Read the model definition and answer for the solid it produces. Units are mm, in the model's axes. Give positions to 0.01 mm unless a question says otherwise; leave off trailing zeros. Loops run counter-clockwise (first coordinate to the right, second up) from the corner with the lowest first, then second, coordinate; pieces in that order, holes last. Notation, with made-up numbers: (21, 3) -> (62, 3) arc R28 ccw to (62, 34) -> close; hole circle Ø8 at (43.25, 77). An arc over 180 degrees is marked (long way). One line per item, written item: value. Start each with the question number.
from build123d import *

# Parameters (mm, degrees)
F0_R     = 10.668
F0_R_2   = 8.255
F1_DEPTH = 914.4
F2_R     = 4.1275
F3_DEPTH = 25.4


with BuildPart() as f1:
    # F0 (on Front) → F1 (new body)
    with BuildSketch(Plane.XZ):
        Circle(F0_R)
        Circle(F0_R_2, mode=Mode.SUBTRACT)
    extrude(amount=F1_DEPTH)

    # F2 (on Top) → F3 (cut)
    with BuildSketch(Plane.XY):
        with Locations((0, -101.6)):
            Circle(F2_R)
        with Locations((0, -279.4)):
            Circle(F2_R)
        with Locations((0, -457.2)):
            Circle(F2_R)
        with Locations((0, -635)):
            Circle(F2_R)
        with Locations((0, -812.8)):
            Circle(F2_R)
    extrude(amount=F3_DEPTH, mode=Mode.SUBTRACT)


solid = f1.part
Item 1: Section C-C, the plane y = -859 is taken. Determine the outline of the cut face in (x, z) (3 decimals), plus the area to 3 significant figures.
Item 2: Section A-A, the plane x = 0 is taken. Determine the outline of the cut face in (y, z) (1 decimal), plus the area to 3 significant figures.
Item 3: Flat-ended cylindrical pins translate along their axes: pin 1 (1 mm diameter, centred on x = -3.5, z = -5.5, fed in from -Y); pin 2 (1 mm diameter, centred on x = 4.5, y = -630.5, fed in from -Z); pin 3 (2 mm diameter, centred on y = -575, z = -8, fed in from +X); pin 4 (1.5 mm diameter, centred on x = 7, y = -187.5, fed in from +Z). Find the tip coordinate at first contact, or state that the pin passes through.
Item 4: Determine the mould class of faces 1 (the cylindrical face through (7.874, -450.799, 2.48)), 2 (the flat face through (3, -914.4, -8)), 3 (the cylindrical face through (4.923, -450.799, -9.464)) for opening direction X: pulls with the +X half, pulls with the -X half, needs draft (parallel to the pull), parting line crosses it, or undercut.
Item 5: Section B-B, the plane z = 3.75 is taken. Determine the outline of the cut face in (x, y).
Item 6: Consider L1, parallel to Y at x = 0, z = 9.8; L2, parallel to Z at x = 1.5, y = -771.5; L3, parallel to X at y = -656, z = 1. Determine where each line is inside the solid, lowest interval first. Write a range as [from, to].
Computed values:
1. outline: circle Ø21.336 at (0, 0); hole circle Ø16.51 at (0, 0)
1. area: 143 mm²
2. outline: (-914.4, -10.7) -> (0, -10.7) -> (0, -8.3) -> (-914.4, -8.3) -> close; (-914.4, 8.3) -> (-816.9, 8.3) -> (-816.9, 10.7) -> (-914.4, 10.7) -> close; (-808.7, 8.3) -> (-639.1, 8.3) -> (-639.1, 10.7) -> (-808.7, 10.7) -> close; (-630.9, 8.3) -> (-461.3, 8.3) -> (-461.3, 10.7) -> (-630.9, 10.7) -> close; (-453.1, 8.3) -> (-283.5, 8.3) -> (-283.5, 10.7) -> (-453.1, 10.7) -> close; (-275.3, 8.3) -> (-105.7, 8.3) -> (-105.7, 10.7) -> (-275.3, 10.7) -> close; (-97.5, 8.3) -> (0, 8.3) -> (0, 10.7) -> (-97.5, 10.7) -> close
2. area: 4,310 mm²
3. pin 1: through
3. pin 2: z = -9.89
3. pin 3: x = 8.05
3. pin 4: z = 8.65
4. face 1: undercut
4. face 2: needs draft
4. face 3: parting line crosses it
5. outline: (-9.99, -914.4) -> (-7.35, -914.4) -> (-7.35, 0) -> (-9.99, 0) -> close; (7.35, -914.4) -> (9.99, -914.4) -> (9.99, 0) -> (7.35, 0) -> close
6. L1: [-914.4, -816.93], [-808.67, -639.13], [-630.87, -461.33], [-453.07, -283.53], [-275.27, -105.73], [-97.47, 0]
6. L2: [-10.56, -8.12], [8.12, 10.56]
6. L3: [-10.62, -8.19], [8.19, 10.62]
